Could you check a few things on this model? Use its own coordinates, in mm. A direction names the side the tool comes from. Coordinates: 2 decimals unless noted, no trailing zeros. Loops run counter-clockwise (first coordinate to the right, second up) from the corner with the lowest first, then second, coordinate; pieces in that order, holes last.
1) Imagine slicing it at A-A on z = -12. Please give me the cut outline in (x, y).
2) Imagine slicing it at D-D on y = 43.5. Please give me the cut outline in (x, z).
3) If I drill on line 1 along Z through (x, y) = (43, 15.5); line 2 along Y through (x, z) = (-49, 33); line 3 along Z through (x, y) = (80, 1), over which ranges is the centre line in solid material (lowest first)?
4) Imagine slicing it at B-B on x = 63. Please give me the cut outline in (y, z), plus the area to 3 significant figures.
5) Imagine slicing it at C-C on x = 2. Please give me the cut outline in (y, z).
6) Thinking about a two-plate mould opening in Y: for faces 1 (the face through (26.856, -10, 25)), 2 (the face through (-9.87, 2.43, 24.23)), 3 (the face through (-96.195, 15, 24)), 4 (the face through (159.706, -19.69, -27.769)), which applies, released by +Y, released by -Y, zero draft, split by the parting line, or undercut?
7) Will these pins go through, and if not, where does the flat tip stop? P1, Ø1.5, axis at y = -9.5, z = 4, coming from the +X side; P2, Ø22.5, axis at x = 96.5, z = 57, coming from the -Y side; P3, Ø8, axis at x = 3.5, z = 68, coming from the +Y side.
8) For faces 5 (the face through (26.856, -51, 24)), 6 (the face through (2, 82, -17.891)), 7 (the face through (134.656, -40, 23)), 8 (the face through (2, 82, 67.891)), which set-ups out of +Z, -Z, +X, -X, +Y, -Y let a thin tool reach every point of the face, with its end or its side?
```python
from build123d import *

# Parameters (mm, degrees)
SKETCH2_R           = 10
BOSS_EXTRUDE1_DEPTH = 50
CUT_EXTRUDE1_DEPTH  = 64.068151531
BOSS_EXTRUDE2_START = 49
BOSS_EXTRUDE2_DEPTH = 49
FILLET1_R           = 10
CHAMFER1_SIZE       = 7.5
CHAMFER1_SIZE2      = 6.781071912
CHAMFER2_SIZE       = 2
CHAMFER3_SIZE       = 2
FILLET2_R           = 2
SCALE1_SCALE        = 2
SCALE2_SCALE        = 1.1
SKETCH5_W           = 159.672226339
SKETCH5_H           = 42.890755139
SKETCH5_H_2         = 42.890755138
BOSS_EXTRUDE3_DEPTH = 3


with BuildPart() as part:
    # Sketch2 → Boss-Extrude1 (new body)
    with BuildSketch(Plane.XY):
        Polygon((40.193713233, 38.980676174), (-42.791413838, 48.363568548), (-42.791413838, -25.22727884), (8.499789264, -25.22727884), (13.140434631, -20.586633473), (13.140434631, -6.901832716), (69.990252121, -6.901832716), (77.208586162, -0.271434231), (77.208586162, 4.980676174), align=None)
        with Locations((-12.791413838, 11.568144854)):
            Circle(SKETCH2_R, mode=Mode.SUBTRACT)
    extrude(amount=BOSS_EXTRUDE1_DEPTH)

    # Sketch3 → Cut-Extrude1 (cut)
    with BuildSketch(Plane(origin=(77.208586162, 0, 0), x_dir=(0, 0, -1), z_dir=(1, 0, 0))):
        with BuildLine():
            Line((-38.573939088, 4.980676174), (-25, 4.980676174))
            Line((-25, 4.980676174), (-11.426060912, 4.980676174))
            ThreePointArc((-11.426060912, 4.980676174), (-25, 16.180248925), (-38.573939088, 4.980676174))
        make_face()
        with BuildLine():
            Line((-38.573939088, -0.271434231), (-25, -0.271434231))
            Line((-25, -0.271434231), (-25, 4.980676174))
            Line((-25, 4.980676174), (-38.573939088, 4.980676174))
            ThreePointArc((-38.573939088, 4.980676174), (-38.825627953, 2.354620972), (-38.573939088, -0.271434231))
        make_face()
        with BuildLine():
            Line((-25, 4.980676174), (-25, -0.271434231))
            Line((-25, -0.271434231), (-11.426060912, -0.271434231))
            ThreePointArc((-11.426060912, -0.271434231), (-11.237438102, 1.035576506), (-11.174372047, 2.354620972))
            ThreePointArc((-11.174372047, 2.354620972), (-11.237438102, 3.673665437), (-11.426060912, 4.980676174))
            Line((-11.426060912, 4.980676174), (-25, 4.980676174))
        make_face()
        with BuildLine():
            Line((-11.426060912, -0.271434231), (-25, -0.271434231))
            Line((-25, -0.271434231), (-38.573939088, -0.271434231))
            ThreePointArc((-38.573939088, -0.271434231), (-25, -11.471006981), (-11.426060912, -0.271434231))
        make_face()
    extrude(amount=-CUT_EXTRUDE1_DEPTH, mode=Mode.SUBTRACT)

    # Sketch4 → Boss-Extrude2 (add)
    with BuildSketch(Plane(origin=(13.140434631, 0, 0), x_dir=(0, 0, -1), z_dir=(1, 0, 0)).offset(BOSS_EXTRUDE2_START)):
        with BuildLine():
            Line((-13.196692619, -6.901832716), (-14.730333334, -6.901832716))
            ThreePointArc((-14.730333334, -6.901832716), (-25, -11.471006981), (-35.269666666, -6.901832716))
            Line((-35.269666666, -6.901832716), (-36.803307381, -6.901832716))
            ThreePointArc((-36.803307381, -6.901832716), (-25, -12.645379028), (-13.196692619, -6.901832716))
        make_face()
    extrude(amount=-BOSS_EXTRUDE2_DEPTH)

    # Fillet1
    fillet1_edges = [part.edges().sort_by_distance(p)[0] for p in [
        (-42.791413838, -25.22727884, 25),
    ]]
    fillet(fillet1_edges, radius=FILLET1_R)

    # Chamfer1
    chamfer1_edges = [part.edges().sort_by_distance(p)[0] for p in [
        (-42.791413838, 48.363568548, 25),
    ]]
    chamfer1_side = [part.faces().sort_by_distance(p)[0] for p in [
        (-1.298850303, 43.672122361, 25),
    ]]
    chamfer(chamfer1_edges, length=CHAMFER1_SIZE, length2=CHAMFER1_SIZE2, reference=chamfer1_side[0])

    # Chamfer2
    chamfer2_edges = [part.edges().sort_by_distance(p)[0] for p in [
        (2.427406766, 43.250805069, 0),
        (58.701149697, 21.980676174, 0),
        (58.701149697, 21.980676174, 50),
        (2.427406766, 43.250805069, 50),
    ]]
    chamfer(chamfer2_edges, length=CHAMFER2_SIZE)

    # Chamfer3
    chamfer3_edges = [part.edges().sort_by_distance(p)[0] for p in [
        (41.565343376, -6.901832716, 50),
        (73.599419141, -3.586633473, 50),
        (73.599419141, -3.586633473, 0),
        (41.565343376, -6.901832716, 0),
    ]]
    chamfer(chamfer3_edges, length=CHAMFER3_SIZE)

    # Fillet2
    fillet2_edges = [part.edges().sort_by_distance(p)[0] for p in [
        (13.140434631, -6.901832716, 7.598346309),
        (13.140434631, -12.645379028, 25),
        (13.140434631, -6.901832716, 42.401653691),
    ]]
    fillet(fillet2_edges, radius=FILLET2_R)


with BuildPart() as part_1:
    # Scale1: scaled about (1.71120361, 12.165140941, 25)
    add(part.part.scale(SCALE1_SCALE).moved(Location((-1.71120361, -12.165140941, -25))))


with BuildPart() as part_2:
    # Scale2: scaled about (1.711203609, 12.165140942, 25)
    add(part_1.part.scale(SCALE2_SCALE).moved(Location((-0.171120361, -1.216514094, -2.5))))

    # Sketch5 → Boss-Extrude3 (add)
    with BuildSketch(Plane(origin=(9.034485149, 79.903708601, 0), x_dir=(0.993668551555422, -0.11235127791774192, 0), z_dir=(0.11235127791774194, 0.9936685515554221, 0))):
        with Locations((-5.784473025, -46.445353997)):
            Rectangle(SKETCH5_W, SKETCH5_H)
        with Locations((-5.784473025, -3.554598859)):
            Rectangle(SKETCH5_W, SKETCH5_H_2)
    extrude(amount=BOSS_EXTRUDE3_DEPTH)


solid = part_2.part
```
Filled in:
1. outline: (-96.19, -48.1) arc R22 ccw to (-74.19, -70.1) - (16.65, -70.1) - (26.86, -59.89) - (26.86, -34.18) arc R4.4 cw to (31.26, -29.78) - (151.93, -29.78) - (167.81, -15.2) - (167.81, -3.64) - (86.37, 71.16) - (82.62, 71.58) - (82.95, 74.56) - (-75.71, 92.5) - (-76.04, 89.52) - (-79.8, 89.95) - (-96.19, 76.88) - close; hole circle Ø44 at (-30.19, 10.85)
2. outline: (-96.19, -30) - (109.98, -30) - (116.48, -25.6) - (116.48, 75.6) - (109.98, 80) - (-96.19, 80) - close
3. line 1: z = -30 to 7.56, 42.44 to 80
3. line 2: y = -70.1 to -0.57, 22.27 to 89.48
3. line 3: z = -30 to -3.58, 53.58 to 80
4. outline: (-29.78, -25.6) - (-25.38, -30) - (69.37, -30) - (73.8, -25.6) - (73.8, -17.89) - (76.82, -17.89) - (76.82, 67.89) - (73.8, 67.89) - (73.8, 75.6) - (69.37, 80) - (-25.38, 80) - (-29.78, 75.6) - (-29.78, 50.97) arc R33 ccw to (-29.78, -0.97) - close; hole circle Ø60.83 at (-9.42, 25)
4. area: 9,170 mm2
5. outline: (-70.1, -30) - (76.27, -30) - (80.7, -25.6) - (80.7, -17.89) - (83.72, -17.89) - (83.72, 67.89) - (80.7, 67.89) - (80.7, 75.6) - (76.27, 80) - (-70.1, 80) - close
6. face 1: undercut
6. face 2: undercut
6. face 3: zero draft
6. face 4: released by -Y
7. P1: stops at x = 26.86
7. P2: stops at y = -35.08
7. P3: stops at y = 84
8. face 5: +X, -Y
8. face 6: -Z, +X, +Y
8. face 7: +Z, -Z, +X, -Y
8. face 8: +Z, +X, +Y
